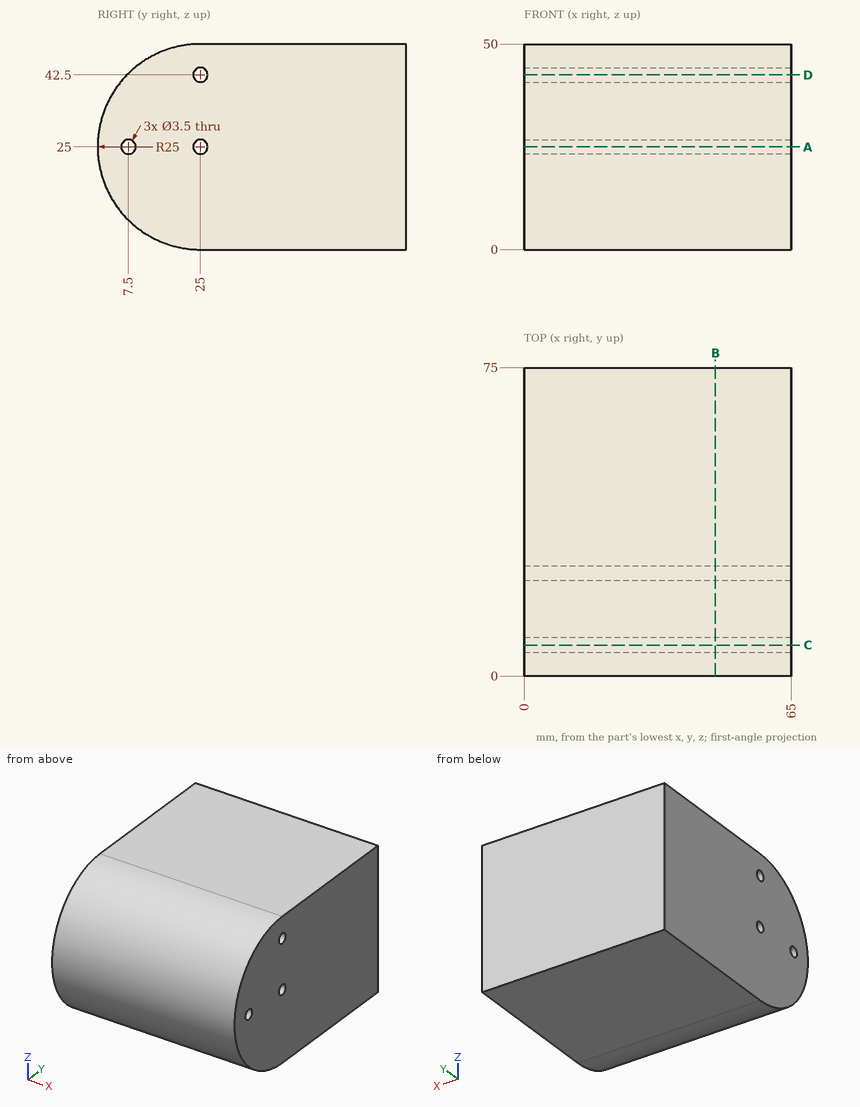
Geometry check sheet. Reference: drawing and pictorial views, mm from the part's lowest x, y, z. Coordinates: 2 decimals unless noted, no trailing zeros. Write each loop counter-clockwise with the first axis right and the second up, starting at its lowest first coordinate (ties: lowest second). Pieces come first, ordered by that corner, then holes. Notation, with made-up numbers: M 2,-11 L 26,-11 A26 ccw 26,28 Z; hole C -25,76.5 d3. An arc over 180 degrees is marked long. Write item = value, one per line. Start each with the question number.
1. Sectioned sample at B-B (x = 46.5). Record the cut outline in (y, z), then the cut area to 3 significant figures.
2. Sectioned sample at D-D (z = 42.5). Record the cut outline in (x, y).
3. Sectioned sample at C-C (y = 7.5). Record the cut outline in (x, z), then the cut area to 3 significant figures.
4. Go/stop test with flat-tipped pins: pin 1 (4 mm diameter, centred on x = 45, z = 40, fed in from -Y); pin 2 (3 mm diameter, centred on y = 7.5, z = 25, fed in from -X); pin 3 (6 mm diameter, centred on x = 9.5, z = 5, fed in from -Y). Record where each tip stops, or that it passes through.
5. Thickness scan on probe 1 along Z at (x, y) = (34, 25); probe 2 along Y at (x, z) = (39, 24.5) (3 decimals); probe 3 along Y at (x, z) = (52, 24). Record the ranges inside material, lowest first.
6. Sectioned sample at A-A (z = 25). Record the cut outline in (x, y).
The answers:
q1.outline = M 25,0 L 75,0 L 75,50 L 25,50 A25 ccw Z; hole C 7.5,25 d3.5; hole C 25,25 d3.5; hole C 25,42.5 d3.5
q1.area = 3,450 mm²
q2.outline = M 0,7.15 L 65,7.15 L 65,23.25 L 0,23.25 Z; M 0,26.75 L 65,26.75 L 65,75 L 0,75 Z
q3.outline = M 0,7.15 L 65,7.15 L 65,23.25 L 0,23.25 Z; M 0,26.75 L 65,26.75 L 65,42.85 L 0,42.85 Z
q3.area = 2,090 mm²
q4.pin_1 = 3.65
q4.pin_2 = through
q4.pin_3 = 6.67
q5.probe_1 = 0 to 23.25, 26.75 to 40.75, 44.25 to 50
q5.probe_2 = 0.005 to 5.823, 9.177 to 23.323, 26.677 to 75
q5.probe_3 = 0.02 to 6.06, 8.94 to 23.56, 26.44 to 75
q6.outline = M 0,0 L 65,0 L 65,5.75 L 0,5.75 Z; M 0,9.25 L 65,9.25 L 65,23.25 L 0,23.25 Z; M 0,26.75 L 65,26.75 L 65,75 L 0,75 Z
